Read the model definition and answer for the solid it produces. Units are mm, in the model's axes. A direction names the side the tool comes from. Coordinates: 2 decimals unless noted, no trailing zeros. Write each loop counter-clockwise with the first axis right and the second up, starting at its lowest first coordinate (ties: lowest second). Pieces come first, ordered by that corner, then holes.
Item 1: Section C-C (z = 15.5) is taken. Give the vertices of the cut face in (x, y) (3 decimals), then the cut area to 3 significant figures.
Item 2: Section B-B (x = 19.05) is taken. Give the vertices of the cut face in (y, z) (3 decimals), then the cut area to 3 significant figures.
Item 3: Section A-A (y = 0) is taken. Give the vertices of the cut face in (x, z) (3 decimals).
Item 4: A tool of negligible diameter and unlimited length cuts with its end or side. For faces 1 (the face through (19, 38.1, 9)), 2 (the face through (12.7, 35, 9)), from which of +Z, -Z, +X, -X, +Y, -Y can it reach the whole face along a straight path? Write none if from no direction.
Item 5: This flat-tipped pin is pushed along its axis until it touches: P1, Ø4, axis at x = 19.05, y = 19.05, coming from the +Z side. Where does it stop, or does it pass through?
Item 6: Section D-D (y = 19.05) is taken. Give the vertices of the cut face in (x, z) (3 decimals), then the cut area to 3 significant figures.
Item 7: Determine the mould class of faces 3 (the face through (-11, 20, 19.05)), 4 (the face through (-11, 20, 0)), 5 (the face through (-16.53, 17.12, 9.39)), 6 (the face through (-19.139, 34.536, 9.665)) for opening direction Z: released by +Z, released by -Z, zero draft, split by the parting line, or undercut.
Item 8: Straight lines are drawn through the part: probe 1 along X at (y, z) = (17.5, 9); probe 2 along Y at (x, z) = (-17, 18); probe 3 along X at (y, z) = (-19.5, 7.75). For each, find the intervals that lie inside material, in ascending order.
from build123d import *

# Parameters (mm, degrees)
SKETCH1_W           = 50.8
SKETCH1_H           = 50.8
BOSS_EXTRUDE1_DEPTH = 19.05
SKETCH2_R           = 22.225
CUT_EXTRUDE1_DEPTH  = 25.4
SKETCH3_W           = 19.05
SKETCH3_H           = 12.7
SKETCH3_R           = 3.175
BOSS_EXTRUDE2_DEPTH = 12.7
SKETCH4_R           = 3.175
CUT_EXTRUDE2_DEPTH  = 50.595085442


with BuildPart() as part:
    # Sketch1 → Boss-Extrude1 (new body)
    with BuildSketch(Plane.XY):
        Rectangle(SKETCH1_W, SKETCH1_H)
    extrude(amount=BOSS_EXTRUDE1_DEPTH)

    # Sketch2 → Cut-Extrude1 (cut)
    with BuildSketch(Plane(origin=(0, 0, 0), x_dir=(-1, 0, 0), z_dir=(0, 0, -1))):
        Circle(SKETCH2_R)
    extrude(amount=-CUT_EXTRUDE1_DEPTH, mode=Mode.SUBTRACT)

    # Sketch3 → Boss-Extrude2 (add)
    with BuildSketch(Plane.ZY.offset(25.4)):
        with Locations((9.525, 31.75)):
            Rectangle(SKETCH3_W, SKETCH3_H)
        with Locations(Location((9.525, 31.363785976, 0), (0, 0, 270))):
            Circle(SKETCH3_R, mode=Mode.SUBTRACT)
    boss_extrude2 = extrude(amount=-BOSS_EXTRUDE2_DEPTH)

    # Mirror1: Boss-Extrude2 across plane
    add(boss_extrude2.mirror(Plane(origin=(0, 0, 0), x_dir=(0, 0, 1), z_dir=(1, 0, 0))))

    # Sketch4 → Cut-Extrude2 (cut, through all)
    with BuildSketch(Plane(origin=(0, 0, 0), x_dir=(-1, 0, 0), z_dir=(0, 0, -1))):
        with Locations((-19.05, 19.05)):
            Circle(SKETCH4_R)
        with Locations((19.05, 19.05)):
            Circle(SKETCH4_R)
        with Locations((19.05, -19.05)):
            Circle(SKETCH4_R)
        with Locations((-19.05, -19.05)):
            Circle(SKETCH4_R)
    extrude(amount=-CUT_EXTRUDE2_DEPTH, mode=Mode.SUBTRACT)


solid = part.part
Established:
1. outline: (-25.4, -25.4) - (25.4, -25.4) - (25.4, 38.1) - (12.7, 38.1) - (12.7, 25.4) - (-12.7, 25.4) - (-12.7, 38.1) - (-25.4, 38.1) - close; hole circle Ø6.35 at (-19.05, -19.05); hole circle Ø44.45 at (0, 0); hole circle Ø6.35 at (-19.05, 19.05); hole circle Ø6.35 at (19.05, -19.05); hole circle Ø6.35 at (19.05, 19.05)
1. area: 1,220 mm2
2. outline: (-25.4, 0) - (-22.225, 0) - (-22.225, 19.05) - (-25.4, 19.05) - close; (-15.875, 0) - (-11.448, 0) - (-11.448, 19.05) - (-15.875, 19.05) - close; (11.448, 0) - (15.875, 0) - (15.875, 19.05) - (11.448, 19.05) - close; (22.225, 0) - (38.1, 0) - (38.1, 19.05) - (22.225, 19.05) - close; hole circle Ø6.35 at (31.364, 9.525)
2. area: 500 mm2
3. outline: (-25.4, 0) - (-22.225, 0) - (-22.225, 19.05) - (-25.4, 19.05) - close; (22.225, 0) - (25.4, 0) - (25.4, 19.05) - (22.225, 19.05) - close
4. face 1: +Z, -Z, +X, -X, +Y
4. face 2: +Z, -Z, +Y
5. P1: passes through
6. outline: (-25.4, 0) - (-22.225, 0) - (-22.225, 19.05) - (-25.4, 19.05) - close; (-15.875, 0) - (-11.448, 0) - (-11.448, 19.05) - (-15.875, 19.05) - close; (11.448, 0) - (15.875, 0) - (15.875, 19.05) - (11.448, 19.05) - close; (22.225, 0) - (25.4, 0) - (25.4, 19.05) - (22.225, 19.05) - close
6. area: 290 mm2
7. face 3: released by +Z
7. face 4: released by -Z
7. face 5: zero draft
7. face 6: undercut
8. probe 1: x = -25.4 to -21.82, -16.28 to -13.7, 13.7 to 16.28, 21.82 to 25.4
8. probe 2: y = -25.4 to -21.47, -16.63 to -14.32, 14.32 to 16.63, 21.47 to 38.1
8. probe 3: x = -25.4 to -22.19, -15.91 to -10.66, 10.66 to 15.91, 22.19 to 25.4
